Autodesk Inventor part; units mm, degrees
ref_plane "Work Plane1" through (0, -48.7997, 0.6985) normal (0, 1, 0) x (1, 0, 0)
ref_plane "Work Plane2" through (0, -50.8, 0.6985) normal (0, -1, 0) x (1, 0, 0)
ref_plane "YZ Plane" through (0, 0, 0) normal (1, 0, 0) x (0, 1, 0)
sketch "Sketch1" plane through (0, 0, 0) normal (0, 0, 1) x (1, 0, 0)
  line L0 (-1.905, -50.8) -> (1.905, -50.8)
  line L1 (1.905, -50.8) -> (1.905, 50.8)
  line L2 (1.905, 50.8) -> (-1.905, 50.8) construction
  line L3 (-1.905, 50.8) -> (-1.905, -50.8)
  line L4 (-1.905, -50.8) -> (1.905, 50.8) construction
  line L5 (1.905, -50.8) -> (-1.905, 50.8) construction
  line L6 (-1.905, 50.8) -> (0, 57.8088)
  line L7 (0, 57.8088) -> (1.905, 50.8)
  line L8 (0, 50.8) -> (0, 57.8088) construction
  point P0 (0, 0)
  dimension "d0" = 3.81
  dimension "d1" = 101.6
extrude "Extrusion1" add sketch "Sketch1" along normal blind 1.397
sketch "Sketch2" plane through (-1.905, -50.8, 0) normal (0, -1, 0) x (1, 0, 0)
  line L0 (0, 0) -> (3.81, 1.397) construction
  line L1 (3.81, 1.397) -> (3.81, 0) construction
  line L2 (3.81, 0) -> (0, 1.397) construction
  circle A0 centre (1.905, 0.6985) radius 3.175
  point P0 (1.905, 0)
  dimension "d4" = 6.35
extrude "Extrusion2" add sketch "Sketch2" against normal blind 4.0005
ref_plane "Work Plane1" through (0, -48.7997, 0.6985) normal (0, 1, 0) x (1, 0, 0)
ref_plane "Work Plane2" through (0, -50.8, 0.6985) normal (0, -1, 0) x (1, 0, 0)
ref_plane "Work Plane3" through (0, 0, 0.6985) normal (0, 0, 1) x (1, 0, 0)
properties part number "Zip tie start"
Model file for the job. Use its own axes, mm. A direction names the side the tool comes from. Give positions to 0.01 mm unless a question says otherwise; leave off trailing zeros. Order: outer loops, then holes, each group sorted by start corner. A loop starts at its lowest first (then second) coordinate and runs counter-clockwise, first axis right, second up. Notation, with made-up numbers: (6, 24) - (46, 24) arc R26 ccw to (46, 48) - close; hole circle Ø2 at (-34, 37.5). An arc over 180 degrees is marked (long way). One line per item, written item: value.
Item 1: Slice it at A-A (y = -20). List the corners of the cut face in (x, z) (3 decimals).
Response values:
outline: (-1.905, 0) - (1.905, 0) - (1.905, 1.397) - (-1.905, 1.397) - close
Item 2: Pin check, flat tips, straight feed: pin 1 Ø1.5 at (x, y) = (1, -26.5) entering from +Z; pin 2 Ø0.7 at (y, z) = (25.5, 1) entering from +X (3 decimals); pin 3 Ø1.1 at (y, z) = (19, 0.5) entering from -X (3 decimals). Stop position of each tip, or through.
Response values:
pin 1: z = 1.4
pin 2: x = 1.905
pin 3: x = -1.905
Item 3: Tool access for faces 1 (the flat face through (0, 6, 1.397)), 2 (the flat face through (0, 6, 0)), 3 (the flat face through (-0.966, 54.255, 0.689)): list every direction of +Z, -Z, +X, -X, +Y, -Y with a clear straight run to the whole face (end or side of a thin tool).
Response values:
face 1: +Z, +X, -X, +Y
face 2: -Z, +X, -X, +Y
face 3: +Z, -Z, -X, +Y
Item 4: Wall check: line 1 (Z direction, x = 1.75, y = 47); line 2 (Y direction, x = -2, z = 1.5); line 3 (X direction, y = 9, z = 1.25) (3 decimals). Give the ranges that are in metal, low to high.
Response values:
line 1: 0 to 1.4
line 2: -50.8 to -46.8
line 3: -1.905 to 1.905
